```python
from build123d import *

# Parameters (mm, degrees)
SKETCH_1_W               = 22.514200142
SKETCH_1_H               = 10.000016773
SKETCH_1_R               = 1.55
SKETCH_1_W_2             = 82
SKETCH_1_H_2             = 20
EXTRUDE_3_DEPTH          = 6
SKETCH_3_W               = 82
SKETCH_3_H               = 20
EXTRUDE_4_DEPTH          = 49
SKETCH_5_R               = 4.1
CUT_EXTRUDE_2_DEPTH      = 15
SKETCH_6_R               = 5.06
CUT_EXTRUDE_3_DEPTH      = 15
CUT_EXTRUDE_4_DEPTH      = 75.87323291
CUT_EXTRUDE_4_DEPTH_BACK = 75.87323291
SKETCH_7_W               = 28.844452319
SKETCH_7_H               = 12
CUT_EXTRUDE_5_DEPTH      = 5


with BuildPart() as part:
    # Эскиз1 → Бобышка-Вытянуть3 (new body)
    # profile 1 of 5: a face of its own
    with BuildSketch(Plane(origin=(0, 0, 0), x_dir=(1, 0, 0), z_dir=(0, 1, 0))):
        with Locations((-29.742899929, 15.000008387)):
            Rectangle(SKETCH_1_W, SKETCH_1_H)
        with Locations(Location((-35.379367801, 15.000008387, 0), (0, 0, 270))):
            Circle(SKETCH_1_R, mode=Mode.SUBTRACT)
        with Locations(Location((-29.739367801, 15.000008387, 0), (0, 0, 270))):
            Circle(SKETCH_1_R, mode=Mode.SUBTRACT)
        with Locations(Location((-24.106432057, 15.000008387, 0), (0, 0, 270))):
            Circle(SKETCH_1_R, mode=Mode.SUBTRACT)
    # profile 2 of 5: a face of its own
    with BuildSketch(Plane(origin=(0, 0, 0), x_dir=(1, 0, 0), z_dir=(0, 1, 0))):
        Rectangle(SKETCH_1_W_2, SKETCH_1_H_2)
    # profile 3 of 5: a face of its own
    with BuildSketch(Plane(origin=(0, 0, 0), x_dir=(1, 0, 0), z_dir=(0, 1, 0))):
        with Locations((-29.742899929, -15.000008387)):
            Rectangle(SKETCH_1_W, SKETCH_1_H)
        with Locations(Location((-35.379367801, -15.000008387, 0), (0, 0, 270))):
            Circle(SKETCH_1_R, mode=Mode.SUBTRACT)
        with Locations(Location((-29.739367801, -15.000008387, 0), (0, 0, 270))):
            Circle(SKETCH_1_R, mode=Mode.SUBTRACT)
        with Locations(Location((-24.106432057, -15.000008387, 0), (0, 0, 270))):
            Circle(SKETCH_1_R, mode=Mode.SUBTRACT)
    # profile 4 of 5: a face of its own
    with BuildSketch(Plane(origin=(0, 0, 0), x_dir=(1, 0, 0), z_dir=(0, 1, 0))):
        with Locations((29.742899929, -15.000008387)):
            Rectangle(SKETCH_1_W, SKETCH_1_H)
        with Locations(Location((24.106432057, -15.000008387, 0), (0, 0, 270))):
            Circle(SKETCH_1_R, mode=Mode.SUBTRACT)
        with Locations(Location((29.739367801, -15.000008387, 0), (0, 0, 270))):
            Circle(SKETCH_1_R, mode=Mode.SUBTRACT)
        with Locations(Location((35.379367801, -15.000008387, 0), (0, 0, 270))):
            Circle(SKETCH_1_R, mode=Mode.SUBTRACT)
    # profile 5 of 5: a face of its own
    with BuildSketch(Plane(origin=(0, 0, 0), x_dir=(1, 0, 0), z_dir=(0, 1, 0))):
        with Locations((29.742899929, 15.000008387)):
            Rectangle(SKETCH_1_W, SKETCH_1_H)
        with Locations(Location((24.106432057, 15.000008387, 0), (0, 0, 270))):
            Circle(SKETCH_1_R, mode=Mode.SUBTRACT)
        with Locations(Location((29.739367801, 15.000008387, 0), (0, 0, 270))):
            Circle(SKETCH_1_R, mode=Mode.SUBTRACT)
        with Locations(Location((35.379367801, 15.000008387, 0), (0, 0, 270))):
            Circle(SKETCH_1_R, mode=Mode.SUBTRACT)
    extrude(amount=EXTRUDE_3_DEPTH)

    # Эскиз3 → Бобышка-Вытянуть4 (add)
    with BuildSketch(Plane(origin=(0, 6, 0), x_dir=(1, 0, 0), z_dir=(0, 1, 0))):
        Rectangle(SKETCH_3_W, SKETCH_3_H)
    extrude(amount=EXTRUDE_4_DEPTH)

    # Эскиз5 → Вырез-Вытянуть2 (cut)
    with BuildSketch(Plane.XY.offset(10)):
        with Locations((32.25, 31.072649375)):
            Circle(SKETCH_5_R)
        with Locations(Location((-32.25, 31.072649375, 0), (0, 0, 180))):
            Circle(SKETCH_5_R)
    extrude(amount=-CUT_EXTRUDE_2_DEPTH, mode=Mode.SUBTRACT)

    # Эскиз6 → Вырез-Вытянуть3 (cut)
    with BuildSketch(Plane.XY.offset(10)):
        with Locations((0.178742266, 31.522649375)):
            Circle(SKETCH_6_R)
    extrude(amount=-CUT_EXTRUDE_3_DEPTH, mode=Mode.SUBTRACT)

    # Эскиз4 → Вырез-Вытянуть4 (cut, two sides: drawn at the far end of the back side and taken through both)
    with BuildSketch(Plane(origin=(0, 0, -10), x_dir=(-1, 0, 0), z_dir=(0, 0, -1)).offset(-CUT_EXTRUDE_4_DEPTH_BACK)):
        Polygon((41, 39), (41, 38.572649375), (-41, 39), (-41, 55), (41, 55), align=None)
    extrude(amount=CUT_EXTRUDE_4_DEPTH + CUT_EXTRUDE_4_DEPTH_BACK, mode=Mode.SUBTRACT)

    # Эскиз7 → Вырез-Вытянуть5 (cut)
    with BuildSketch(Plane.XY.offset(10)):
        with Locations((0.061520834, 18.208477718)):
            Rectangle(SKETCH_7_W, SKETCH_7_H)
    extrude(amount=-CUT_EXTRUDE_5_DEPTH, mode=Mode.SUBTRACT)


solid = part.part
```
For this review, take the finished solid that the model builds, in its own axes (mm). A direction names the side the tool comes from. Coordinates: 2 decimals unless noted, no trailing zeros. Loops run counter-clockwise (first coordinate to the right, second up) from the corner with the lowest first, then second, coordinate; pieces in that order, holes last. Notation, with made-up numbers: (-17, -40) - (41, -40) arc R23 ccw to (41, -18) - close; hole circle Ø5 at (13, 12). An arc over 180 degrees is marked (long way). Use one line per item in the form item = value. Start each with the question number.
1) To check wall thickness, follow probe 1 along X at (y, z) = (23, 7.5); probe 2 along Z at (x, y) = (-12.5, 4); probe 3 along Y at (x, z) = (29.5, 6.5). State the ranges of each line that lie inside material, in increasing order. Write a range as from..to.
2) For pin 1 (11 mm diameter, centred on x = -32.5, z = -17, fed in from +Y); pin 2 (3.5 mm diameter, centred on x = 1, y = 16, fed in from +Z); pin 3 (5 mm diameter, centred on x = -7.5, y = 6.5, fed in from +Z); pin 4 (5.5 mm diameter, centred on x = 3, z = 6.5, fed in from -Y), all flat-tipped, find the tip position at first contact; note any pin that passes through.
3) Take a section at C-C (z = 2). State the section outline as (x, y) points.
4) Take a section at A-A (z = -11.5). State the section outline as (x, y) points.
5) Draft analysis for pull direction X (two halves, no side actions). For faces 6 (the face through (41, 19, 0)), 7 (the face through (18.486, 3, 15)), 8 (the face through (-41, 19, 0)), state which applies: released by +X, released by -X, zero draft, split by the parting line, or undercut.
6) Take a section at D-D (x = 20). State the section outline as (y, z) points, plus the area to 3 significant figures.
7) Take a section at B-B (y = 16.5). State the section outline as (x, z) points.
8) For faces 1 (the face through (0, 32, -5)), 2 (the face through (-30, 6, 13)), 3 (the face through (-18.486, 3, 15)), 4 (the face through (30, 3, -20)), 5 (the face through (18.486, 3, -15)), list the 3-axis set-ups (+Z, -Z, +X, -X, +Y, -Y) from which the entire face can be reached by the end or side of a thin tool; tool diameter is ignored.
From the geometry:
q1.probe_1 = -41..-14.36, 14.48..41
q1.probe_2 = -10..10
q1.probe_3 = 0..28.03, 34.11..38.94
q2.pin_1 = 6
q2.pin_2 = 5
q2.pin_3 = 10
q2.pin_4 = 0
q3.outline = (-41, 0) - (41, 0) - (41, 39) - (-41, 38.57) - close; hole circle Ø8.2 at (-32.25, 31.07); hole circle Ø10.12 at (0.18, 31.52); hole circle Ø8.2 at (32.25, 31.07)
q4.outline = (-41, 0) - (-18.49, 0) - (-18.49, 6) - (-41, 6) - close; (18.49, 0) - (41, 0) - (41, 6) - (18.49, 6) - close
q5.face_6 = released by +X
q5.face_7 = undercut
q5.face_8 = released by -X
q6.outline = (0, -20) - (6, -20) - (6, -10) - (38.89, -10) - (38.89, 10) - (6, 10) - (6, 20) - (0, 20) - close
q6.area = 898 mm2
q7.outline = (-41, -10) - (41, -10) - (41, 10) - (14.48, 10) - (14.48, 5) - (-14.36, 5) - (-14.36, 10) - (-41, 10) - close
q8.face_1 = +Z
q8.face_2 = +Z, +X, -X, +Y
q8.face_3 = +Z, +Y, -Y
q8.face_4 = -Z, +X, -X, +Y, -Y
q8.face_5 = -Z, +Y, -Y
